Verification items for this drawing (mm, ordinates from the low corner). A direction names the side the tool comes from. Round coordinates to 2 decimals unless told otherwise and drop trailing zeros. Loops run counter-clockwise (first coordinate to the right, second up) from the corner with the lowest first, then second, coordinate; pieces in that order, holes last. Notation, with made-up numbers: M -19,84.5 L -15,84.5 A23 ccw -15,120.5 Z; hole C 22.5,21.5 d1. An arc over 180 degrees is marked long. Write item = value, one per line. Start each with the question number.
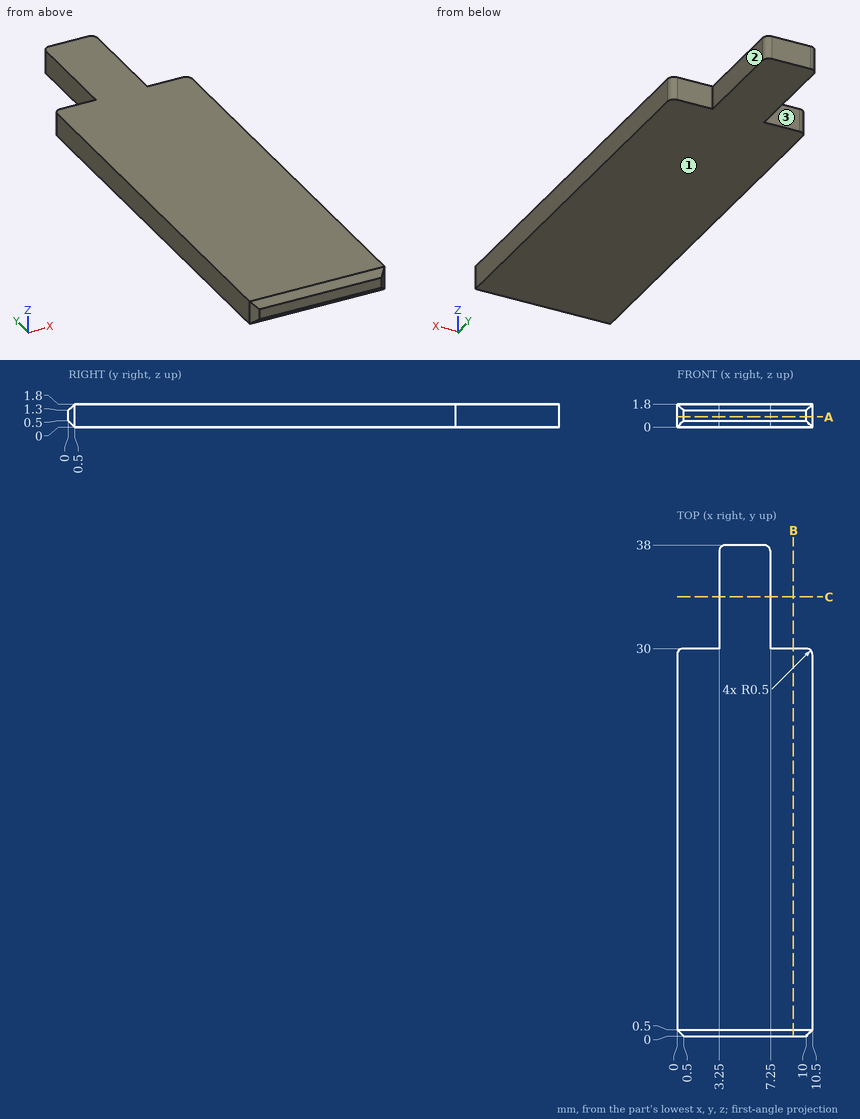
1. Section check A-A, the plane z = 0.8. Enter the section's corners in (x, y), and give its area (3 significant figures).
2. Tool access check on the marked faces 1, 2 and 3. Record the directions out of +Z, -Z, +X, -X, +Y, -Y that give a thin tool (end or side, any length) a straight path to the whole face; none if there is none.
3. Section check B-B, the plane x = 9. Enter the section's corners in (y, z), and give its area (4 significant figures).
4. Gauge pin test, flat ends, axial feed: P1, Ø0.9, axis at y = 34, z = 1, coming from the +X side; P2, Ø0.9, axis at x = 2.5, z = 1.5, coming from the +Y side. Record the tip position at first contact, or that the pin passes through.
5. Section check C-C, the plane y = 34. Enter the section's corners in (x, z).
6. Thickness scan on line 1 (Y direction, x = 2, z = 0.8); line 2 (X direction, y = 32, z = 1.75); line 3 (Y direction, x = 8, z = 1.65). Record the ranges inside material, lowest first.
Computed values:
q1.outline = M 0,0.5 L 0.5,0 L 10,0 L 10.5,0.5 L 10.5,29.5 A0.5 ccw 10,30 L 7.25,30 L 7.25,37.5 A0.5 ccw 6.75,38 L 3.75,38 A0.5 ccw 3.25,37.5 L 3.25,30 L 0.5,30 A0.5 ccw 0,29.5 Z
q1.area = 347 mm2
q2.face_1 = -Z, +X, -X, +Y, -Y
q2.face_2 = +Z, -Z, +X, +Y
q2.face_3 = +Z, -Z, -X, +Y
q3.outline = M 0,0.5 L 0.5,0 L 30,0 L 30,1.8 L 0.5,1.8 L 0,1.3 Z
q3.area = 53.75 mm2
q4.P1 = 7.25
q4.P2 = 30
q5.outline = M 3.25,0 L 7.25,0 L 7.25,1.8 L 3.25,1.8 Z
q6.line_1 = 0 to 30
q6.line_2 = 3.25 to 7.25
q6.line_3 = 0.35 to 30
